from build123d import *

# Parameters (mm, degrees)
F0_W        = 63.5
F0_H        = 247.65
F1_DEPTH    = 1.778
F2_W        = 63.5
F2_H        = 2.54
F3_DEPTH    = 12.7
F4_W        = 14.478
F4_H        = 247.65
F5_DEPTH    = 1.778
F6_W        = 42.672
F6_H        = 76.2
F7_DEPTH    = 12.7
F8_R        = 12.7
F9_R        = 12.7
F10_C1_SIZE = 1.524
F10_C2_SIZE = 1.524
F10_C3_SIZE = 1.5236


# Not quite as in the source:
# - a fillet or chamfer is up to 0.001 mm smaller than in the source, because OpenCascade refuses the exact size


with BuildPart() as f1:
    # F0 (on Front) → F1 (new body)
    with BuildSketch(Plane.XZ):
        with Locations((31.75, 123.825)):
            Rectangle(F0_W, F0_H)
    extrude(amount=F1_DEPTH)

    # F2 (on face) → F3 (join)
    with BuildSketch(Plane.XZ.offset(1.778)):
        with Locations((31.75, 1.27)):
            Rectangle(F2_W, F2_H)
    extrude(amount=F3_DEPTH)

    # F4 (on face) → F5 (join)
    with BuildSketch(Plane.YZ.offset(63.5)):
        with Locations((-7.239, 123.825)):
            Rectangle(F4_W, F4_H)
    extrude(amount=F5_DEPTH)

    # F6 (on face) → F7 (join)
    with BuildSketch(Plane(origin=(0, 0, 0), x_dir=(-1, 0, 0), z_dir=(0, 1, 0))):
        with Locations((-43.942, 12.7)):
            Rectangle(F6_W, F6_H)
    extrude(amount=F7_DEPTH)

    # F8
    f8_edges = [f1.edges().sort_by_distance(p)[0] for p in [
        (0, -0.889, 247.65),
        (64.389, -14.478, 247.65),
    ]]
    fillet(f8_edges, radius=F8_R)

    # F9
    f9_edges = [f1.edges().sort_by_distance(p)[0] for p in [
        (0, -14.478, 1.27),
    ]]
    fillet(f9_edges, radius=F9_R)

    # F10: chamfer of 1.524 on 3 edges, made by hand

    # F10_c1
    f10_c1_edges = [f1.edges().sort_by_distance(p)[0] for p in [
        (0, -1.778, 118.745),
        (3.7197438789, -1.778, 243.9302561211),
        (38.1, -1.778, 247.65),
    ]]
    chamfer(f10_c1_edges, length=F10_C1_SIZE)

    # F10_c2
    f10_c2_edges = [f1.edges().sort_by_distance(p)[0] for p in [
        (3.7197438789, -10.7582561211, 2.54),
        (38.1, -14.478, 2.54),
    ]]
    chamfer(f10_c2_edges, length=F10_C2_SIZE)

    # F10_c3 (size 1.524 in the source; OpenCascade refuses exactly that, so slightly less here)
    f10_c3_edges = [f1.edges().sort_by_distance(p)[0] for p in [
        (63.5, -14.478, 118.745),
        (63.5, -10.7582561211, 243.9302561211),
    ]]
    chamfer(f10_c3_edges, length=F10_C3_SIZE)


solid = f1.part
Geometry check sheet. Reference: the model listing, model coordinates, mm. A direction names the side the tool comes from. Round coordinates to 2 decimals unless told otherwise and drop trailing zeros. Write each loop counter-clockwise with the first axis right and the second up, starting at its lowest first coordinate (ties: lowest second). Pieces come first, ordered by that corner, then holes. Notation, with made-up numbers: (-21, -0.5) - (-16, -0.5) arc R4 cw to (-16, 3.5) - close; hole circle Ø6 at (69.5, -35). An arc over 180 degrees is marked (long way). One line per item, written item: value.
1. Mould release check, pull along Y, two halves, no side actions. Record for faces 1 (the face through (65.278, -4, 109)), 2 (the face through (44, 12.7, 13)), 3 (the face through (32, -1.778, 126)): released by +Y, released by -Y, zero draft, split by the parting line, or undercut.
The answers:
face 1: zero draft
face 2: released by +Y
face 3: released by -Y
2. Cross-section at A-A on x = 57.5. Record the boundary of the cut face in (y, z).
The answers:
outline: (-14.48, 0) - (0, 0) - (0, -25.4) - (12.7, -25.4) - (12.7, 50.8) - (0, 50.8) - (0, 247.65) - (-0.25, 247.65) - (-1.78, 246.13) - (-1.78, 2.54) - (-12.95, 2.54) - (-14.48, 1.02) - close
3. Cross-section at B-B on z = 27. Record the boundary of the cut face in (x, y).
The answers:
outline: (0, -0.25) - (1.52, -1.78) - (63.5, -1.78) - (63.5, -12.95) - (65.02, -14.48) - (65.28, -14.48) - (65.28, 12.7) - (22.61, 12.7) - (22.61, 0) - (0, 0) - close
4. Scan lines: L1, parallel to Z at x = 60.5, y = -12.25; L2, parallel to Y at x = 28.5, z = 50; L3, parallel to X at y = -7.75, z = 23. Record each from-to range of solid material in increasing order.
The answers:
L1: z = 0 to 2.54
L2: y = -1.78 to 12.7
L3: x = 63.5 to 65.28
5. Depth check by flat-ended pin: pin 1 Ø5.5 at (y, z) = (-8, 155) entering from -X; pin 2 Ø7.5 at (x, z) = (41, -7.5) entering from -Y; pin 3 Ø4 at (x, y) = (55.5, -3.5) entering from +Z. Enter the tip coordinate at first touch or a pass-through.
The answers:
pin 1: stops at x = 63.5
pin 2: stops at y = 0
pin 3: stops at z = 246.4
6. Cross-section at D-D on x = 17.5. Record the boundary of the cut face in (y, z), and give its area (3 significant figures).
The answers:
outline: (-14.48, 0) - (0, 0) - (0, 247.65) - (-0.25, 247.65) - (-1.78, 246.13) - (-1.78, 2.54) - (-12.95, 2.54) - (-14.48, 1.02) - close
area: 470 mm^2
7. Cross-section at C-C on y = 8.5. Record the boundary of the cut face in (x, z).
The answers:
outline: (22.61, -25.4) - (65.28, -25.4) - (65.28, 50.8) - (22.61, 50.8) - close
8. Set-up check for faces 4 (the face through (32, -7, 2.54)), 5 (the face through (22.606, 6, 12)), 6 (the face through (32, -7, 0)): record each of +Z, -Z, +X, -X, +Y, -Y from which the full face is reachable in a straight line by a thin tool's end or side.
The answers:
face 4: +Z, -X, -Y
face 5: +Z, -Z, -X, +Y
face 6: -Z, +X, -X, -Y
